Geometry check sheet. Reference: the model listing, model coordinates, mm. Round coordinates to 2 decimals unless told otherwise and drop trailing zeros. Write each loop counter-clockwise with the first axis right and the second up, starting at its lowest first coordinate (ties: lowest second). Pieces come first, ordered by that corner, then holes. Notation, with made-up numbers: M -4.5,-4.5 L 19.5,-4.5 A22 cw 19.5,2.5 Z; hole C -15.5,31 d7. An arc over 180 degrees is marked long. Use a Markdown table: item, result.
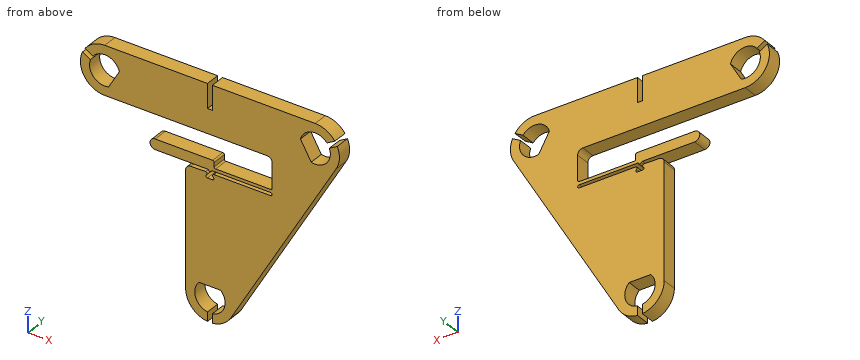
```python
from build123d import *

# Parameters (mm, degrees)
BOSS_EXTRUDE1_DEPTH = 2.4


with BuildPart() as part:
    # Sketch1 → Boss-Extrude1 (new body)
    with BuildSketch(Plane(origin=(0, 0, 0), x_dir=(1, 0, 0), z_dir=(0, 1, 0))):
        with BuildLine():
            Line((-1.767766953, 18.232233047), (1.767766953, 18.232233047))
            ThreePointArc((1.767766953, 18.232233047), (2.379032248, 20.768248374), (0.4, 22.467792536))
            Line((0.4, 22.467792536), (0.4, 23.979949748))
            ThreePointArc((0.4, 23.979949748), (2.170914686, 23.359632335), (3.464101615, 22))
            Line((3.464101615, 22), (20.784609691, -8))
            ThreePointArc((20.784609691, -8), (21.315492368, -9.7997489), (20.967245664, -11.643564713))
            Line((20.967245664, -11.643564713), (19.657679103, -10.887486106))
            ThreePointArc((19.657679103, -10.887486106), (19.175346808, -8.323821824), (16.673460463, -7.585185434))
            Line((16.673460463, -7.585185434), (14.90569351, -10.647047613))
            ThreePointArc((14.90569351, -10.647047613), (16.79631456, -12.44442655), (19.257679103, -11.580306429))
            Line((19.257679103, -11.580306429), (20.567245664, -12.336385036))
            ThreePointArc((20.567245664, -12.336385036), (19.144577682, -13.559883435), (17.320508076, -14))
            Line((17.320508076, -14), (0.4, -14))
            Line((0.4, -14), (0.4, -10))
            Line((0.4, -10), (-0.4, -10))
            Line((-0.4, -10), (-0.4, -14))
            Line((-0.4, -14), (-17.320508076, -14))
            ThreePointArc((-17.320508076, -14), (-19.144577682, -13.559883435), (-20.567245664, -12.336385036))
            Line((-20.567245664, -12.336385036), (-19.257679103, -11.580306429))
            ThreePointArc((-19.257679103, -11.580306429), (-16.79631456, -12.44442655), (-14.90569351, -10.647047613))
            Line((-14.90569351, -10.647047613), (-16.673460463, -7.585185434))
            ThreePointArc((-16.673460463, -7.585185434), (-19.175346808, -8.323821824), (-19.657679103, -10.887486106))
            Line((-19.657679103, -10.887486106), (-20.967245664, -11.643564713))
            ThreePointArc((-20.967245664, -11.643564713), (-20.680140411, -7.829085314), (-17.320508076, -6))
            Line((-17.320508076, -6), (9.396838839, -6))
            ThreePointArc((9.396838839, -6), (10.000114881, -5.750114881), (10.25, -5.146838839))
            Line((10.25, -5.146838839), (10.25, -1.085))
            ThreePointArc((10.25, -1.085), (10.176776695, -0.908223305), (10, -0.835))
            Line((10, -0.835), (0.94831677, -0.835))
            ThreePointArc((0.94831677, -0.835), (0.771540074, -0.908223305), (0.69831677, -1.085))
            Line((0.69831677, -1.085), (0.69831677, -1.791322322))
            ThreePointArc((0.69831677, -1.791322322), (0.625093465, -1.968099017), (0.44831677, -2.041322322))
            Line((0.44831677, -2.041322322), (-9, -2.041322322))
            ThreePointArc((-9, -2.041322322), (-9.853161161, -1.188161161), (-9, -0.335))
            Line((-9, -0.335), (-0.433012702, -0.335))
            ThreePointArc((-0.433012702, -0.335), (-0.308012702, -0.301506351), (-0.216506351, -0.21))
            ThreePointArc((-0.216506351, -0.21), (0, -0.085), (0.216506351, -0.21))
            ThreePointArc((0.216506351, -0.21), (0.308012702, -0.301506351), (0.433012702, -0.335))
            Line((0.433012702, -0.335), (10, -0.335))
            ThreePointArc((10, -0.335), (10.25, -0.085), (10, 0.165))
            Line((10, 0.165), (0.69831677, 0.165))
            ThreePointArc((0.69831677, 0.165), (0.459762847, 0.340220149), (0.555604555, 0.620263791))
            ThreePointArc((0.555604555, 0.620263791), (0.651446263, 0.900307433), (0.412892341, 1.075527582))
            Line((0.412892341, 1.075527582), (-0.412892341, 1.075527582))
            ThreePointArc((-0.412892341, 1.075527582), (-0.651446263, 0.900307433), (-0.555604555, 0.620263791))
            ThreePointArc((-0.555604555, 0.620263791), (-0.460652433, 0.337439296), (-0.704155623, 0.165068194))
            Line((-0.704155623, 0.165068194), (-3.166764771, 0.222599142))
            ThreePointArc((-3.166764771, 0.222599142), (-3.757119102, 0.479338042), (-4, 1.075527582))
            Line((-4, 1.075527582), (-4, 20))
            ThreePointArc((-4, 20), (-2.966479395, 22.683281573), (-0.4, 23.979949748))
            Line((-0.4, 23.979949748), (-0.4, 22.467792536))
            ThreePointArc((-0.4, 22.467792536), (-2.379032248, 20.768248374), (-1.767766953, 18.232233047))
        make_face()
    extrude(amount=BOSS_EXTRUDE1_DEPTH)


solid = part.part
```
Item 1: Go/stop test with flat-tipped pins: pin 1 (0.6 mm diameter, centred on x = 0, y = 1, fed in from +Z); pin 2 (1.2 mm diameter, centred on y = 0.5, z = -23.5, fed in from -X) (3 decimals); pin 3 (1.2 mm diameter, centred on x = 7, y = 0.5, fed in from -Z). Record where each tip stops, or that it passes through.
Outcome:
| item | result |
|---|---|
| pin 1 | stops at z = 10 |
| pin 2 | stops at x = -2.755 |
| pin 3 | stops at z = -16.91 |
Item 2: Cross-section at A-A, the plane x = -8. Record the cut outline in (y, z) (3 decimals).
Outcome:
| item | result |
|---|---|
| outline | M 0,0.335 L 2.4,0.335 L 2.4,2.041 L 0,2.041 Z; M 0,6 L 2.4,6 L 2.4,14 L 0,14 Z |
Item 3: Material ranges on line 1 along Z through (x, y) = (-8.5, 0.65) (3 decimals); line 2 along Z through (x, y) = (4, 0.8) (3 decimals); line 3 along Z through (x, y) = (-3, 1.55) (3 decimals), recorded low to high. Write a range as from..to.
Outcome:
| item | result |
|---|---|
| line 1 | z = 0.335..2.041, 6..14 |
| line 2 | z = -21.072..-0.165, 0.335..0.835, 6..14 |
| line 3 | z = -22.646..-0.219, 0.335..2.041, 6..14 |
Item 4: Cross-section at B-B, the plane x = 5. Record the cut outline in (y, z) (3 decimals).
Outcome:
| item | result |
|---|---|
| outline | M 0,-19.34 L 2.4,-19.34 L 2.4,-0.165 L 0,-0.165 Z; M 0,0.335 L 2.4,0.335 L 2.4,0.835 L 0,0.835 Z; M 0,6 L 2.4,6 L 2.4,14 L 0,14 Z |
Item 5: Cross-section at C-C, the plane x = -13. Record the cut outline in (y, z), and give its area (3 significant figures).
Outcome:
| item | result |
|---|---|
| outline | M 0,6 L 2.4,6 L 2.4,14 L 0,14 Z |
| area | 19.2 mm2 |
